The model under review builds one solid part; all positions refer to its coordinate system, in mm. A direction names the side the tool comes from. Coordinates: 2 decimals unless noted, no trailing zeros. Loops run counter-clockwise (first coordinate to the right, second up) from the corner with the lowest first, then second, coordinate; pieces in that order, holes last. Notation, with made-up numbers: M -33.75,60.5 L 22.25,60.5 A17 ccw 22.25,77.5 Z; hole C 71.5,83 d5. An arc over 180 degrees is marked long. One line per item, written item: value.
```python
from build123d import *

# Parameters (mm, degrees)
SKETCH_2_W               = 2
SKETCH_2_H               = 31.418584287
PATTERN_CIRCULAR_1_COUNT = 2
PATTERN_CIRCULAR_1_ANGLE = 120
CHAMFER_1_SIZE           = 0.2
CHAMFER_2_SIZE           = 0.5


with BuildPart() as part:
    # 草图1 → 旋转1 (revolve)
    with BuildSketch(Plane(origin=(0, 0, 0), x_dir=(0, 0, -1), z_dir=(1, 0, 0)), mode=Mode.PRIVATE) as revolve_1_sk:
        with BuildLine():
            Line((0.861588836, 5), (16.861588836, 5))
            Line((16.861588836, 5), (16.861588836, 10))
            Line((16.861588836, 10), (6.861588836, 10))
            Line((6.861588836, 10), (6.861588836, 23))
            Line((6.861588836, 23), (5.761588836, 23))
            ThreePointArc((5.761588836, 23), (4.011588836, 21.25), (2.261588836, 23))
            Line((2.261588836, 23), (0.861588836, 23))
            Line((0.861588836, 23), (0.861588836, 5))
        make_face()
    revolve(revolve_1_sk.sketch.rotate(Axis((0, 0, 0), (0, 0, -1)), 90), axis=Axis((0, 0, 0), (0, 0, -1)))

    # 草图2 → M4 螺纹孔1 (revolve, cut)
    with BuildSketch(Plane(origin=(0, 0, -12), x_dir=(0, 0, -1), z_dir=(1, 0, 0))):
        with Locations((1, 15.709292144)):
            Rectangle(SKETCH_2_W, SKETCH_2_H)
    hole_wizard_m4_1 = revolve(axis=Axis((0, -6.35, -12), (0, 1, 0)), mode=Mode.SUBTRACT)

    # 阵列(圆周)1: M4 螺纹孔1 ×2 about axis
    pattern_circular_1_axis = Axis((0, 0, 0), (0, 0, 1))
    for i in range(1, PATTERN_CIRCULAR_1_COUNT):
        add(hole_wizard_m4_1.rotate(pattern_circular_1_axis, i * PATTERN_CIRCULAR_1_ANGLE / (PATTERN_CIRCULAR_1_COUNT - 1)), mode=Mode.SUBTRACT)

    # 倒角1
    chamfer_1_edges = [part.edges().sort_by_distance(p)[0] for p in [
        (-23, 0, -0.861588836),
        (-23, 0, -6.861588836),
        (-10, 0, -16.861588836),
        (-5, 0, -16.861588836),
        (-5, 0, -0.861588836),
    ]]
    chamfer(chamfer_1_edges, length=CHAMFER_1_SIZE)

    # 倒角2
    chamfer_2_edges = [part.edges().sort_by_distance(p)[0] for p in [
        (-10, 0, -6.861588836),
    ]]
    chamfer(chamfer_2_edges, length=CHAMFER_2_SIZE)


solid = part.part
```
(1) Add section D-D on z = -4. State the section outline as (x, y) points.
Checks:
outline: C 0,0 d42.5; hole C 0,0 d10
(2) Draft analysis for pull direction Z (two halves, no side actions). For faces 1 (the face through (-2.994, -22.804, -1.653)), 2 (the face through (-6.3, -3.7, -10)), 3 (the face through (-5.4, -0.3, -0.862)), state which applies: pulls with the +Z half, pulls with the -Z half, needs draft (parallel to the pull), parting line crosses it, or undercut.
Checks:
face 1: needs draft
face 2: undercut
face 3: pulls with the +Z half
(3) Add section C-C on z = -12. State the section outline as (x, y) points, then the cut area to 3 significant figures.
Checks:
outline: M -9.49,-3.17 L -4.97,-0.56 A5 cw -2,4.58 L -2,9.8 A10 ccw Z; M -7.49,-6.63 A10 ccw long 2,9.8 L 2,4.58 A5 cw long -2.97,-4.02 Z
area: 195 mm^2
(4) Tool access review of faces 4 (the face through (-4, 4, -16.862)), 5 (the face through (0, 7, -10)), 6 (the face through (-10, 0, -12)): name each direction out of +Z, -Z, +X, -X, +Y, -Y from which nothing blocks a thin tool from reaching the whole face with its end or side.
Checks:
face 4: -Z, +X, -X, +Y, -Y
face 5: +Y
face 6: -Z
(5) Add section B-B on y = 0. State the section outline as (x, z) points, then the cut area to 3 significant figures.
Checks:
outline: M -23,-6.66 L -22.8,-6.86 L -10.5,-6.86 L -10,-7.36 L -10,-16.66 L -9.8,-16.86 L -5.2,-16.86 L -5,-16.66 L -5,-1.06 L -5.2,-0.86 L -22.8,-0.86 L -23,-1.06 L -23,-2.26 A1.75 cw -23,-5.76 Z; M 5,-16.66 L 5.2,-16.86 L 9.8,-16.86 L 10,-16.66 L 10,-7.36 L 10.5,-6.86 L 22.8,-6.86 L 23,-6.66 L 23,-5.76 A1.75 cw 23,-2.26 L 23,-1.06 L 22.8,-0.86 L 5.2,-0.86 L 5,-1.06 Z
area: 306 mm^2
(6) To check wall thickness, follow L1, parallel to Y at x = 0, z = -6.5; L2, parallel to Y at x = 0, z = -7.5; L3, parallel to Z at x = 0, y = 6.55. State the ranges of each line that lie inside material, in increasing order. Write a range as [from, to].
Checks:
L1: [-23, -5], [5, 23]
L2: [-10, -5], [5, 10]
L3: [-16.86, -14], [-10, -0.86]
(7) Insertion check: pin 1 Ø13.5 at (x, y) = (-11, 3) entering from -Z; pin 2 Ø1.5 at (y, z) = (-2, -11.5) entering from -X; pin 3 Ø4 at (y, z) = (8.5, -9) entering from +X; pin 4 Ø4 at (y, z) = (-5.5, -8.5) entering from +X. Each pin has a flat end and moves straight along its axis. Give the tip position at first contact, or say it passes through.
Checks:
pin 1: z = -16.86
pin 2: x = -9.92
pin 3: x = 7.6
pin 4: x = 22.51
(8) Add section A-A on x = 0. State how many separate pieces and enclosed holes the cut face has, then the cut area to 3 significant figures.
Checks:
separate pieces: 3
enclosed holes: 0
area: 286 mm^2
